```python
from build123d import *

# Parameters (mm, degrees)
F0_W     = 3
F0_H     = 58.5
F0_W_2   = 58.5
F0_H_2   = 3
F1_DEPTH = 1


with BuildPart() as f1:
    # F0 (on Top) → F1 (new body, symmetric)
    with BuildSketch(Plane.XY):
        Polygon((-5, 60), (-1.5, 60), (1.5, 60), (5, 60), (5, 70), (-5, 70), align=None)
        with BuildLine():
            ThreePointArc((-2, 61), (-3, 62), (-2, 63))
            ThreePointArc((-2, 63), (-1.2928932188, 62.7071067812), (-1, 62))
            ThreePointArc((-1, 62), (-1.2928932188, 61.2928932188), (-2, 61))
        make_face(mode=Mode.SUBTRACT)
        with BuildLine():
            ThreePointArc((2, 61), (1, 62), (2, 63))
            ThreePointArc((2, 63), (2.7071067812, 62.7071067812), (3, 62))
            ThreePointArc((3, 62), (2.7071067812, 61.2928932188), (2, 61))
        make_face(mode=Mode.SUBTRACT)
        with BuildLine():
            ThreePointArc((2, 64), (1, 65), (2, 66))
            ThreePointArc((2, 66), (2.7071067812, 65.7071067812), (3, 65))
            ThreePointArc((3, 65), (2.7071067812, 64.2928932188), (2, 64))
        make_face(mode=Mode.SUBTRACT)
        with BuildLine():
            ThreePointArc((-2, 69), (-1.2928932188, 68.7071067812), (-1, 68))
            ThreePointArc((-1, 68), (-1.2928932188, 67.2928932188), (-2, 67))
            ThreePointArc((-2, 67), (-3, 68), (-2, 69))
        make_face(mode=Mode.SUBTRACT)
        with BuildLine():
            ThreePointArc((2, 69), (2.7071067812, 68.7071067812), (3, 68))
            ThreePointArc((3, 68), (2.7071067812, 67.2928932188), (2, 67))
            ThreePointArc((2, 67), (1, 68), (2, 69))
        make_face(mode=Mode.SUBTRACT)
        with Locations((0, 30.75)):
            Rectangle(F0_W, F0_H)
        with Locations((30.75, 0)):
            Rectangle(F0_W_2, F0_H_2)
        with Locations((-30.75, 0)):
            Rectangle(F0_W_2, F0_H_2)
        Polygon((60, 5), (60, 1.5), (60, -1.5), (60, -5), (63.5, -5), (66.5, -5), (70, -5), (70, 5), align=None)
        with Locations((0, -30.75)):
            Rectangle(F0_W, F0_H)
        Rectangle(F0_W, F0_H_2)
        with BuildLine():
            ThreePointArc((-1, 62), (-1.2928932188, 62.7071067812), (-2, 63))
            Line((-2, 63), (-2, 61))
            ThreePointArc((-2, 61), (-1.2928932188, 61.2928932188), (-1, 62))
        make_face()
        with BuildLine():
            Line((-2, 61), (-2, 63))
            ThreePointArc((-2, 63), (-3, 62), (-2, 61))
        make_face()
        with BuildLine():
            ThreePointArc((3, 62), (2.7071067812, 62.7071067812), (2, 63))
            Line((2, 63), (2, 61))
            ThreePointArc((2, 61), (2.7071067812, 61.2928932188), (3, 62))
        make_face()
        with BuildLine():
            Line((2, 61), (2, 63))
            ThreePointArc((2, 63), (1, 62), (2, 61))
        make_face()
        with BuildLine():
            Line((-2, 67), (-2, 69))
            ThreePointArc((-2, 69), (-3, 68), (-2, 67))
        make_face()
        with BuildLine():
            ThreePointArc((-2, 67), (-1.2928932188, 67.2928932188), (-1, 68))
            ThreePointArc((-1, 68), (-1.2928932188, 68.7071067812), (-2, 69))
            Line((-2, 69), (-2, 67))
        make_face()
        with BuildLine():
            ThreePointArc((3, 65), (2.7071067812, 65.7071067812), (2, 66))
            Line((2, 66), (2, 64))
            ThreePointArc((2, 64), (2.7071067812, 64.2928932188), (3, 65))
        make_face()
        with BuildLine():
            Line((2, 64), (2, 66))
            ThreePointArc((2, 66), (1, 65), (2, 64))
        make_face()
        with BuildLine():
            Line((2, 67), (2, 69))
            ThreePointArc((2, 69), (1, 68), (2, 67))
        make_face()
        with BuildLine():
            ThreePointArc((2, 67), (2.7071067812, 67.2928932188), (3, 68))
            ThreePointArc((3, 68), (2.7071067812, 68.7071067812), (2, 69))
            Line((2, 69), (2, 67))
        make_face()
    extrude(amount=F1_DEPTH, both=True)

    # F2 (on face) → F3 (revolve)
    with BuildSketch(Plane.XY.offset(1)):
        with BuildLine():
            Line((-2.000000095, 67), (-2.000000095, 69))
            ThreePointArc((-2.000000095, 69), (-3.000000095, 68), (-2.000000095, 67))
        make_face()
        with BuildLine():
            ThreePointArc((-1.000000095, 62), (-1.2928933138, 62.7071067812), (-2.000000095, 63))
            Line((-2.000000095, 63), (-2.000000095, 61))
            ThreePointArc((-2.000000095, 61), (-1.2928933138, 61.2928932188), (-1.000000095, 62))
        make_face()
    revolve(axis=Axis((-2.000000095, 65, 1), (0, -1, 0)))

    # F2 (on face) → F4 (revolve)
    with BuildSketch(Plane.XY.offset(1)):
        with BuildLine():
            ThreePointArc((1.999999905, 67), (2.7071066862, 67.2928932188), (2.999999905, 68))
            ThreePointArc((2.999999905, 68), (2.7071066862, 68.7071067812), (1.999999905, 69))
            Line((1.999999905, 69), (1.999999905, 67))
        make_face()
        with BuildLine():
            Line((1.999999905, 64), (1.999999905, 66))
            ThreePointArc((1.999999905, 66), (0.999999905, 65), (1.999999905, 64))
        make_face()
        with BuildLine():
            Line((1.999999905, 61), (1.999999905, 63))
            ThreePointArc((1.999999905, 63), (0.999999905, 62), (1.999999905, 61))
        make_face()
    revolve(axis=Axis((1.999999905, 65, 1), (0, -1, 0)))

    # F2 (on face) → F5 (revolve)
    with BuildSketch(Plane.XY.offset(1)):
        with BuildLine():
            Line((63, 2), (63, 4))
            ThreePointArc((63, 4), (62, 3), (63, 2))
        make_face()
        with BuildLine():
            ThreePointArc((64, -3), (63.7071067812, -2.2928932188), (63, -2))
            Line((63, -2), (63, -4))
            ThreePointArc((63, -4), (63.7071067812, -3.7071067812), (64, -3))
        make_face()
    revolve(axis=Axis((63, 0, 1), (0, -1, 0)))

    # F2 (on face) → F6 (revolve)
    with BuildSketch(Plane.XY.offset(1)):
        with BuildLine():
            ThreePointArc((67, 2), (67.7071067812, 2.2928932188), (68, 3))
            ThreePointArc((68, 3), (67.7071067812, 3.7071067812), (67, 4))
            Line((67, 4), (67, 2))
        make_face()
        with BuildLine():
            Line((67, -4), (67, -2))
            ThreePointArc((67, -2), (66, -3), (67, -4))
        make_face()
    revolve(axis=Axis((67, 0, 1), (0, -1, 0)))


solid = f1.part
```
For this review, take the finished solid that the model builds, in its own axes (mm). Round coordinates to 2 decimals unless told otherwise and drop trailing zeros. Order: outer loops, then holes, each group sorted by start corner. A loop starts at its lowest first (then second) coordinate and runs counter-clockwise, first axis right, second up.
Q1. Wall thickness on line 1 (X direction, y = -2.5, z = 0.7); line 2 (X direction, y = 34.5, z = -0.3): over which ranges is each line inside the solid? List them lowest first.
Findings below:
line 1: x = -1.5 to 1.5, 60 to 70
line 2: x = -1.5 to 1.5
Q2. We need section B-B, the plane y = 17. Give the boundary of the cut face in (x, z).
Findings below:
outline: (-1.5, -1) - (1.5, -1) - (1.5, 1) - (-1.5, 1) - close
Q3. We need section A-A, the plane z = 0.2. Give the boundary of the cut face in (x, y).
Findings below:
outline: (-60, -1.5) - (-1.5, -1.5) - (-1.5, -60) - (1.5, -60) - (1.5, -1.5) - (60, -1.5) - (60, -5) - (70, -5) - (70, 5) - (60, 5) - (60, 1.5) - (1.5, 1.5) - (1.5, 60) - (5, 60) - (5, 70) - (-5, 70) - (-5, 60) - (-1.5, 60) - (-1.5, 1.5) - (-60, 1.5) - close
Q4. Insertion check: P1, Ø0.6, axis at x = 65, z = 0, coming from the +Y side; P2, Ø1.6, axis at x = -2.5, z = -0.5, coming from the -Y side; P3, Ø1.6, axis at y = 63.5, z = 0, coming from the +X side; P4, Ø6, axis at x = 5.5, y = -5, coming from the -Z side. Each pin has a flat end and moves straight along its axis. Give the tip position at first contact, or say it passes through.
Findings below:
P1: stops at y = 5
P2: stops at y = -1.5
P3: stops at x = 5
P4: passes through
